from build123d import *

# Parameters (mm, degrees)
SKETCH1_W               = 30
SKETCH1_H               = 70
SKETCH1_W_2             = 15
SKETCH1_H_2             = 10
BOSS_EXTRUDE1_DEPTH     = 10
CHAMFER1_SIZE           = 5
CUT_EXTRUDE1_DEPTH      = 213
SKETCH3_R               = 2.1
CUT_EXTRUDE2_DEPTH      = 213
CUT_EXTRUDE3_DEPTH      = 213
CUT_EXTRUDE3_DEPTH_BACK = 4.1
SKETCH4_R               = 3.6


with BuildPart() as part:
    # Sketch1 → Boss-Extrude1 (new body)
    with BuildSketch(Plane.XY):
        with Locations((0, 40)):
            Rectangle(SKETCH1_W, SKETCH1_H)
        with Locations((22.5, 0)):
            Rectangle(SKETCH1_W_2, SKETCH1_H_2)
        Rectangle(SKETCH1_W, SKETCH1_H_2)
        with Locations((-22.5, 0)):
            Rectangle(SKETCH1_W_2, SKETCH1_H_2)
    extrude(amount=BOSS_EXTRUDE1_DEPTH)

    # Chamfer1
    chamfer1_edges = [part.edges().sort_by_distance(p)[0] for p in [
        (-15, 75, 5),
        (15, 75, 5),
        (15, 5, 5),
        (30, 5, 5),
        (-30, 5, 5),
        (-15, 5, 5),
    ]]
    chamfer(chamfer1_edges, length=CHAMFER1_SIZE)

    # Sketch2 → Cut-Extrude1 (cut)
    with BuildSketch(Plane(origin=(0, 75, 0), x_dir=(1, 0, 0), z_dir=(0, 1, 0))):
        Polygon((7.500239939, -7), (-7.500239939, -7), (-3.5, 0), (3.5, 0), align=None)
    extrude(amount=-CUT_EXTRUDE1_DEPTH, mode=Mode.SUBTRACT)

    # Sketch3 → Cut-Extrude2 (cut)
    with BuildSketch(Plane(origin=(0, 5, 0), x_dir=(1, 0, 0), z_dir=(0, 1, 0))):
        with Locations(Location((22.5, -5, 0), (0, 0, 180))):
            Circle(SKETCH3_R)
        with Locations((-22.5, -5)):
            Circle(SKETCH3_R)
    extrude(amount=-CUT_EXTRUDE2_DEPTH, mode=Mode.SUBTRACT)

    # Sketch4 → Cut-Extrude3 (cut, two sides: drawn at the far end of the back side and taken through both)
    with BuildSketch(Plane(origin=(0, 5, 0), x_dir=(1, 0, 0), z_dir=(0, 1, 0)).offset(-CUT_EXTRUDE3_DEPTH_BACK)):
        with Locations(Location((22.5, -5, 0), (0, 0, 46.01703687))):
            Circle(SKETCH4_R)
        with Locations((-22.5, -5)):
            Circle(SKETCH4_R)
    extrude(amount=CUT_EXTRUDE3_DEPTH + CUT_EXTRUDE3_DEPTH_BACK, mode=Mode.SUBTRACT)


solid = part.part
Geometry check sheet. Reference: the model listing, model coordinates, mm. A direction names the side the tool comes from. Coordinates: 2 decimals unless noted, no trailing zeros. Order: outer loops, then holes, each group sorted by start corner. A loop starts at its lowest first (then second) coordinate and runs counter-clockwise, first axis right, second up. Notation, with made-up numbers: (26, 29) - (78, 29) arc R21 cw to (78, 64) - close; hole circle Ø3 at (24.5, 1.5). An arc over 180 degrees is marked (long way). One line per item, written item: value.
(1) Sectioned sample at C-C (y = 49). Enter the section's corners in (x, z), and give its area (3 significant figures).
Data:
outline: (-15, 0) - (-3.5, 0) - (-7.5, 7) - (7.5, 7) - (3.5, 0) - (15, 0) - (15, 10) - (-15, 10) - close
area: 223 mm^2
(2) Thickness scan on probe 1 along Z at (x, y) = (-22.5, 2); probe 2 along Z at (x, y) = (-0.5, 2); probe 3 along Y at (x, z) = (17.5, 2.25). Record the ranges inside material, lowest first. Write a range as from..to.
Data:
probe 1: z = 0..1.4, 8.6..10
probe 2: z = 7..10
probe 3: y = -5..7.5
(3) Sectioned sample at D-D (x = -1.5). Enter the section's corners in (y, z).
Data:
outline: (-5, 7) - (75, 7) - (75, 10) - (-5, 10) - close
(4) Access from +Z, -Z, +X, -X, +Y, -Y to the whole of each face (thin tool, end or side, straight path). Record for faces 4 (the face through (-21, 0.9, 7)), 5 (the face through (-23, 5, 1)), 6 (the face through (5.5, 35.6, 3.5)).
Data:
face 4: +Y
face 5: +Z, -Z, -X, +Y
face 6: +Y, -Y
(5) Depth check by flat-ended pin: pin 1 Ø1.9 at (x, z) = (-22.5, 8.5) entering from +Y; pin 2 Ø6 at (x, z) = (22, 4) entering from +Y; pin 3 Ø2 at (y, z) = (45, 8.5) entering from +X. Enter the tip coordinate at first touch or a pass-through.
Data:
pin 1: stops at y = 5
pin 2: stops at y = 6
pin 3: stops at x = 15
(6) Sectioned sample at B-B (z = 5). Count the separate pieces of the cut face and the enclosed holes in it, and give its area (3 significant figures).
Data:
separate pieces: 4
enclosed holes: 0
area: 1,550 mm^2
(7) Release check for a two-part mould opening along Z. For faces 1 (the face through (-5.5, 35.6, 3.5)), 2 (the face through (-23, 5, 9)), 3 (the face through (11, 36, 0)) record: +Z half, -Z half, draft (parallel to the pull), parting line (faces both ways), or undercut.
Data:
face 1: undercut
face 2: draft
face 3: -Z half
(8) Sectioned sample at A-A (x = 22.5). Enter the section's corners in (y, z).
Data:
outline: (-5, 0) - (5, 0) - (5, 1.4) - (0.9, 1.4) - (0.9, 2.9) - (-5, 2.9) - close; (-5, 7.1) - (0.9, 7.1) - (0.9, 8.6) - (5, 8.6) - (5, 10) - (-5, 10) - close
